Read the model definition and answer for the solid it produces. Units are mm, in the model's axes. Face numbers are marked on the shaded views. Give positions to 0.01 mm unless a question says otherwise; leave off trailing zeros. Order: outer loops, then holes, each group sorted by start corner. A loop starts at its lowest first (then second) coordinate and runs counter-clockwise, first axis right, second up. Notation, with made-up numbers: (80.5, 54) - (91.5, 54) arc R12 cw to (91.5, 67) - close; hole circle Ø1 at (68, 2). An arc over 180 degrees is marked (long way). Write each question's results on one line, items separated by ' | '. Start each with the question number.
Q1. Find section D-D on z = -7.75. Give the vertices of the cut face in (x, y).
Q2. Find section A-A on z = 0. Give the vertices of the cut face in (x, y) (3 decimals).
Q3. For a pull along Y with two mould halves and no side action, classify the marked faces 1, 2 and 3 as +Y half, -Y half, draft (parallel to the pull), parting line (faces both ways), or undercut.
Q4. Find section C-C on x = 1.5. Give the vertices of the cut face in (y, z) (3 decimals).
Q5. Flat-ended cylindrical pins translate along their axes: P1, Ø10, axis at y = 0, z = 0, coming from the -X side; P2, Ø3, axis at x = -1, y = -4.5, coming from the -Z side. Find the tip coordinate at first contact, or state that the pin passes through.
Q6. Find the intervals of material crossed by line 1 along Y through (x, z) = (5.25, -2) (3 decimals); line 2 along Z through (x, y) = (-2.75, 0.5); line 3 along Z through (x, y) = (2, -3.5), in increasing order. Write a range as from..to.
Q7. Find section B-B on y = -2. Give the vertices of the cut face in (x, z), and give its area (3 significant figures).
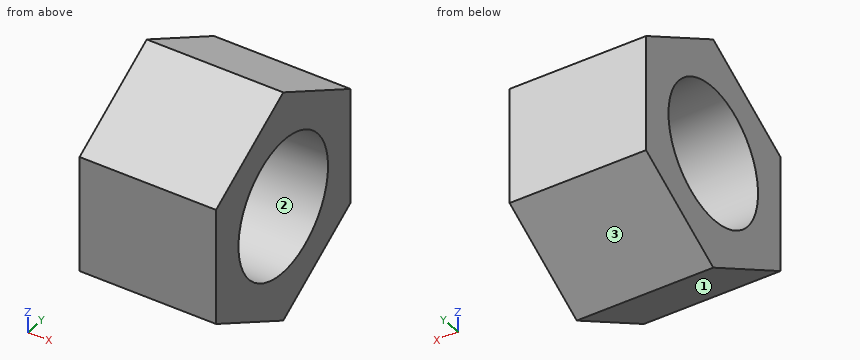
from build123d import *

# Parameters (mm, degrees)
F1_DEPTH = 6.35
F2_R     = 6.35
F3_DEPTH = 12.7


with BuildPart() as f1:
    # F0 (on Right) → F1 (new body, symmetric)
    with BuildSketch(Plane.YZ):
        Polygon((9.525, -5.499261), (9.525, 5.499261), (0, 10.998523), (-9.525, 5.499261), (-9.525, -5.499261), (0, -10.998523), align=None)
    extrude(amount=F1_DEPTH, both=True)

    # F2 (on face) → F3 (cut, symmetric)
    with BuildSketch(Plane.YZ.offset(6.35)):
        Circle(F2_R)
    extrude(amount=F3_DEPTH, both=True, mode=Mode.SUBTRACT)


solid = f1.part
Working result:
1) outline: (-6.35, -5.63) - (6.35, -5.63) - (6.35, 5.63) - (-6.35, 5.63) - close
2) outline: (-6.35, -9.525) - (6.35, -9.525) - (6.35, -6.35) - (-6.35, -6.35) - close; (-6.35, 6.35) - (6.35, 6.35) - (6.35, 9.525) - (-6.35, 9.525) - close
3) face 1: -Y half | face 2: undercut | face 3: +Y half
4) outline: (-9.525, -5.499) - (0, -10.999) - (9.525, -5.499) - (9.525, 5.499) - (0, 10.999) - (-9.525, 5.499) - close; hole circle Ø12.7 at (0, 0)
5) P1: through | P2: z = -9.27
6) line 1: -9.525..-6.027, 6.027..9.525 | line 2: -10.71..-6.33, 6.33..10.71 | line 3: -8.98..-5.3, 5.3..8.98
7) outline: (-6.35, -9.84) - (6.35, -9.84) - (6.35, -6.03) - (-6.35, -6.03) - close; (-6.35, 6.03) - (6.35, 6.03) - (6.35, 9.84) - (-6.35, 9.84) - close | area: 97.0 mm²
